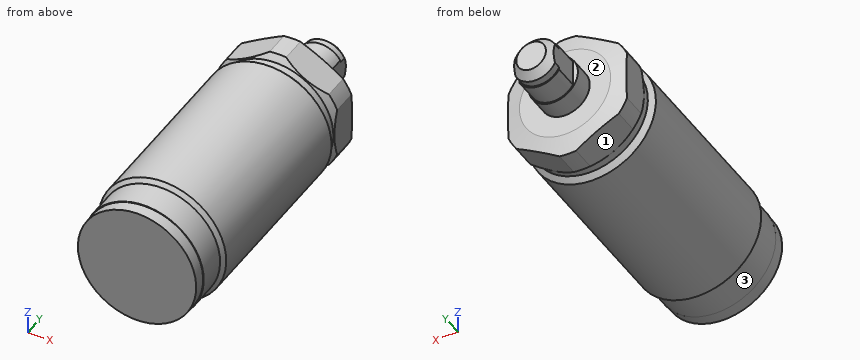
```python
from build123d import *

# Parameters (mm, degrees)
SKETCH1_R          = 13
STOCK_DEPTH        = 27.25
HEX_HEAD_DEPTH     = 8.5
SKETCH5_R          = 12
RETAINER_DEPTH     = 2.5
SKETCH9_W          = 0.724432229
SKETCH9_H          = 3.174333178
SKETCH9_W_2        = 8
SKETCH9_H_2        = 0.600364256
SKETCH9_W_3        = 0.732916959
CUT_EXTRUDE3_DEPTH = 13.475
SKETCH10_R         = 5
EXTRUDE4_DEPTH     = 9.25
SKETCH13_R         = 5
SKETCH13_R_2       = 4.75
CUT_EXTRUDE4_DEPTH = 5
SKETCH14_W         = 1
SKETCH14_H         = 5
CUT_EXTRUDE5_DEPTH = 13.475


with BuildPart() as part:
    # Sketch1 → STOCK (new body, symmetric)
    with BuildSketch(Plane(origin=(0, 0, 0), x_dir=(1, 0, 0), z_dir=(0, 1, 0))):
        with Locations(Location((0, 0, 0), (0, 0, 270))):  # turned: the seam where the file's is
            Circle(SKETCH1_R)
    extrude(amount=STOCK_DEPTH, both=True)

    # Sketch2 → HEX_HEAD (cut)
    with BuildSketch(Plane(origin=(0, 27.25, 0), x_dir=(1, 0, 0), z_dir=(0, 1, 0))):
        with BuildLine():
            ThreePointArc((10.330127019, 7.892304845), (6.5, 11.258330249), (1.669872981, 12.892304845))
            Line((1.669872981, 12.892304845), (10.330127019, 7.892304845))
        make_face()
        with BuildLine():
            Line((-10.330127019, 7.892304845), (-1.669872981, 12.892304845))
            ThreePointArc((-1.669872981, 12.892304845), (-6.5, 11.258330249), (-10.330127019, 7.892304845))
        make_face()
        with BuildLine():
            Line((12, 5), (12, -5))
            ThreePointArc((12, -5), (13, 0), (12, 5))
        make_face()
        with BuildLine():
            Line((-12, -5), (-12, 5))
            ThreePointArc((-12, 5), (-13, 0), (-12, -5))
        make_face()
        with BuildLine():
            Line((10.330127019, -7.892304845), (1.669872981, -12.892304845))
            ThreePointArc((1.669872981, -12.892304845), (6.5, -11.258330249), (10.330127019, -7.892304845))
        make_face()
        with BuildLine():
            Line((-1.669872981, -12.892304845), (-10.330127019, -7.892304845))
            ThreePointArc((-10.330127019, -7.892304845), (-6.5, -11.258330249), (-1.669872981, -12.892304845))
        make_face()
    extrude(amount=-HEX_HEAD_DEPTH, mode=Mode.SUBTRACT)

    # Sketch3 → CROWN (revolve, cut)
    with BuildSketch(Plane.XY, mode=Mode.PRIVATE) as crown_sk:
        Polygon((9.25, 27.25), (13, 27.25), (13, 26.245190528), align=None)
    revolve(crown_sk.sketch.rotate(Axis((0, 0, 0), (0, 1, 0)), 97.380135052), axis=Axis((0, 0, 0), (0, 1, 0)), mode=Mode.SUBTRACT)  # turned: the seam where the file's is

    # Sketch4 → OD_PROFILE (revolve, cut)
    with BuildSketch(Plane.XY, mode=Mode.PRIVATE) as od_profile_sk:
        Polygon((17.017319953, -27.25), (17.017319953, 25.142319953), (11.875, 20), (11.875, 18.5), (12.925, 17.45), (12.925, -20.56), (12.125, -21.36), (12.125, -27.25), align=None)
    revolve(od_profile_sk.sketch.rotate(Axis((0, -29.172938247, 0), (0, 1, 0)), 90), axis=Axis((0, -29.172938247, 0), (0, 1, 0)), mode=Mode.SUBTRACT)  # turned: the seam where the file's is

    # Sketch5 → RETAINER (add)
    with BuildSketch(Plane.XZ.offset(27.25)):
        with Locations(Location((0, 0, 0), (0, 0, 90))):  # turned: the seam where the file's is
            Circle(SKETCH5_R)
    extrude(amount=RETAINER_DEPTH)



with BuildPart() as body_2:
    # Sketch8 → Revolve1 (revolve)
    with BuildSketch(Plane.XY, mode=Mode.PRIVATE) as revolve1_sk:
        Polygon((0, 39.5), (3, 39.5), (4.5, 38), (4.5, 36.5), (0, 36.5), align=None)
    revolve(revolve1_sk.sketch.rotate(Axis((0, 0, 0), (0, 1, 0)), 90), axis=Axis((0, 0, 0), (0, 1, 0)))  # turned: the seam where the file's is

    # Sketch9 → Cut-Extrude3 (cut, symmetric)
    with BuildSketch(Plane.XY):
        with Locations((4.362216115, 38.087166589)):
            Rectangle(SKETCH9_W, SKETCH9_H)
        with Locations((0, 36.199817872)):
            Rectangle(SKETCH9_W_2, SKETCH9_H_2)
        with Locations((-4.36645848, 38.087166589)):
            Rectangle(SKETCH9_W_3, SKETCH9_H)
    extrude(amount=CUT_EXTRUDE3_DEPTH, both=True, mode=Mode.SUBTRACT)


with BuildPart() as part_1:
    add(part.part)

    add(body_2.part)  # Extrude4 merges body 2
    # Sketch10 → Extrude4 (add)
    with BuildSketch(Plane(origin=(0, 27.25, 0), x_dir=(1, 0, 0), z_dir=(0, 1, 0))):
        with Locations(Location((0, 0, 0), (0, 0, 180))):  # turned: the seam where the file's is
            Circle(SKETCH10_R)
    extrude(amount=EXTRUDE4_DEPTH)

    # Sketch13 → Cut-Extrude4 (cut)
    with BuildSketch(Plane(origin=(0, 36.5, 0), x_dir=(1, 0, 0), z_dir=(0, 1, 0))):
        with Locations(Location((0, 0, 0), (0, 0, 180))):  # turned: the seam where the file's is
            Circle(SKETCH13_R)
        with Locations(Location((0, 0, 0), (0, 0, 180))):  # turned: the seam where the file's is
            Circle(SKETCH13_R_2, mode=Mode.SUBTRACT)
    extrude(amount=-CUT_EXTRUDE4_DEPTH, mode=Mode.SUBTRACT)

    # Sketch14 → Cut-Extrude5 (cut, symmetric)
    with BuildSketch(Plane.XY):
        with Locations((4.5, 34)):
            Rectangle(SKETCH14_W, SKETCH14_H)
        with Locations((-4.5, 34)):
            Rectangle(SKETCH14_W, SKETCH14_H)
    extrude(amount=CUT_EXTRUDE5_DEPTH, both=True, mode=Mode.SUBTRACT)


solid = part_1.part
```
The listing builds one solid part. Answer for the finished solid, in the listing's coordinates (mm). Face numbers are marked on the shaded views. A direction names the side the tool comes from. Give positions to 0.01 mm unless a question says otherwise; leave off trailing zeros. Order: outer loops, then holes, each group sorted by start corner. A loop starts at its lowest first (then second) coordinate and runs counter-clockwise, first axis right, second up. Notation, with made-up numbers: (-38.5, -22.5) - (10.5, -22.5) arc R5 cw to (10.5, -17.5) - close; hole circle Ø6 at (61, -8.5). An arc over 180 degrees is marked (long way). Answer in a Markdown table with one row per item. Add a question column.
Q1. Find the intervals of material crossed by line 1 along Y through (x, z) = (1, -8); line 2 along Z through (x, y) = (-7.75, -20); line 3 along Z through (x, y) = (-0.75, 0.5), in increasing order. Write a range as [from, to].
Q2. Which of the six approach directions +Z, -Z, +X, -X, +Y, -Y give full straight-line access (tool end or side, diameter ignored) to the marked faces 1, 2 and 3?
Q3. Given P1, Ø3, axis at x = 0.5, z = 4, coming from the +Y side; P2, Ø4, axis at x = -5, y = 24, coming from the +Z side; P3, Ø1, axis at y = 30, z = -3, coming from the +X side; P4, Ø5, axis at x = -8, y = -12, coming from the +Z side, each flat-ended and moving along its own axis, determine where each tip first touches the part or whether it passes through.
Q4. The part is cut by section B-B (y = 9.5). Determine the outline of the cut face in (x, z) (3 decimals).
Determined:
| question | item | result |
|---|---|---|
| 1 | line 1 | y = [-29.75, 27.25] |
| 1 | line 2 | z = [-10.34, 10.34] |
| 1 | line 3 | z = [-12.9, 12.9] |
| 2 | face 1 | -Z, -X, +Y |
| 2 | face 2 | +Y |
| 2 | face 3 | -Y |
| 3 | P1 | stops at y = 39.5 |
| 3 | P2 | stops at z = 12.12 |
| 3 | P3 | stops at x = 4.33 |
| 3 | P4 | stops at z = 11.7 |
| 4 | outline | circle Ø25.85 at (0, 0) |
